from build123d import *

# Parameters (mm, degrees)
SKETCH1_R             = 12.7
BOSS_EXTRUDE1_DEPTH   = 4.7625
SKETCH2_R             = 7.9375
BOSS_EXTRUDE2_DEPTH   = 6.35
F_4_CLEARANCE_HOLE1_D = 4.7625


with BuildPart() as part:
    # Sketch1 → Boss-Extrude1 (new body)
    with BuildSketch(Plane(origin=(0, 0, 0), x_dir=(0, 0, -1), z_dir=(1, 0, 0))):
        with Locations(Location((0, 0, 0), (0, 0, 180))):
            Circle(SKETCH1_R)
    extrude(amount=BOSS_EXTRUDE1_DEPTH)

    # Sketch2 → Boss-Extrude2 (add)
    with BuildSketch(Plane.ZY):
        with Locations(Location((0, 0, 0), (0, 0, 180))):
            Circle(SKETCH2_R)
    extrude(amount=BOSS_EXTRUDE2_DEPTH)

    # #4 Clearance Hole1 (through all)
    with Locations(Plane(origin=(4.7625, 0, 0), x_dir=(0, 0, -1), z_dir=(1, 0, 0))):
        with Locations((0, 0)):
            Hole(F_4_CLEARANCE_HOLE1_D / 2)


solid = part.part
Geometry check sheet. Reference: the model listing, model coordinates, mm. A direction names the side the tool comes from. Coordinates: 2 decimals unless noted, no trailing zeros. Order: outer loops, then holes, each group sorted by start corner. A loop starts at its lowest first (then second) coordinate and runs counter-clockwise, first axis right, second up. Notation, with made-up numbers: (42, 6) -> (67, 6) arc R24 ccw to (67, 25) -> close; hole circle Ø9 at (-33, 38.25). An arc over 180 degrees is marked (long way). Use a Markdown table: item, result. Add a question column.
1. Cross-section at D-D (z = -3.5). Enter the section's corners in (x, y).
2. Material ranges on L1, parallel to Y at x = -4, z = 0; L2, parallel to Y at x = 2.25, z = 0; L3, parallel to Z at x = -2, y = 2, recorded low to high.
3. Cross-section at C-C (x = 3.25). Enter the section's corners in (y, z), and give its area (3 significant figures).
4. Mould release check, pull along Y, two halves, no side actions. Record for faces 1 (the face through (-0.87, -1.45, -1.89)), 2 (the face through (0, 8.3, -0.2)), 3 (the face through (2.348, 11.267, 5.86)): pulls with the +Y half, pulls with the -Y half, needs draft (parallel to the pull), parting line crosses it, or undercut.
5. Cross-section at A-A (z = 0). Enter the section's corners in (x, y), and give its area (3 significant figures).
6. Go/stop test with flat-tipped pins: pin 1 Ø1 at (x, y) = (-3, 2) entering from -Z; pin 2 Ø3 at (x, z) = (1, -8.5) entering from -Y; pin 3 Ø3 at (x, y) = (-3, -7.5) entering from -Z; pin 4 Ø2 at (y, z) = (1, 0) entering from +X. Record where each tip stops, or that it passes through.
7. Set-up check for faces 4 (the face through (-3.13, 7.75, 1.72)), 5 (the face through (4.762, 0, 3)): record each of +Z, -Z, +X, -X, +Y, -Y from which the full face is reachable in a straight line by a thin tool's end or side.
Filled sheet:
| question | item | result |
|---|---|---|
| 1 | outline | (-6.35, -7.12) -> (0, -7.12) -> (0, -12.21) -> (4.76, -12.21) -> (4.76, 12.21) -> (0, 12.21) -> (0, 7.12) -> (-6.35, 7.12) -> close |
| 2 | L1 | -7.94 to -2.38, 2.38 to 7.94 |
| 2 | L2 | -12.7 to -2.38, 2.38 to 12.7 |
| 2 | L3 | -7.68 to -1.29, 1.29 to 7.68 |
| 3 | outline | circle Ø25.4 at (0, 0); hole circle Ø4.76 at (0, 0) |
| 3 | area | 489 mm2 |
| 4 | face 1 | undercut |
| 4 | face 2 | needs draft |
| 4 | face 3 | parting line crosses it |
| 5 | outline | (-6.35, -7.94) -> (0, -7.94) -> (0, -12.7) -> (4.76, -12.7) -> (4.76, -2.38) -> (-6.35, -2.38) -> close; (-6.35, 2.38) -> (4.76, 2.38) -> (4.76, 12.7) -> (0, 12.7) -> (0, 7.94) -> (-6.35, 7.94) -> close |
| 5 | area | 169 mm2 |
| 6 | pin 1 | z = -7.79 |
| 6 | pin 2 | y = -10.6 |
| 6 | pin 3 | z = -5.2 |
| 6 | pin 4 | through |
| 7 | face 4 | -X |
| 7 | face 5 | +Z, -Z, +X, +Y, -Y |
